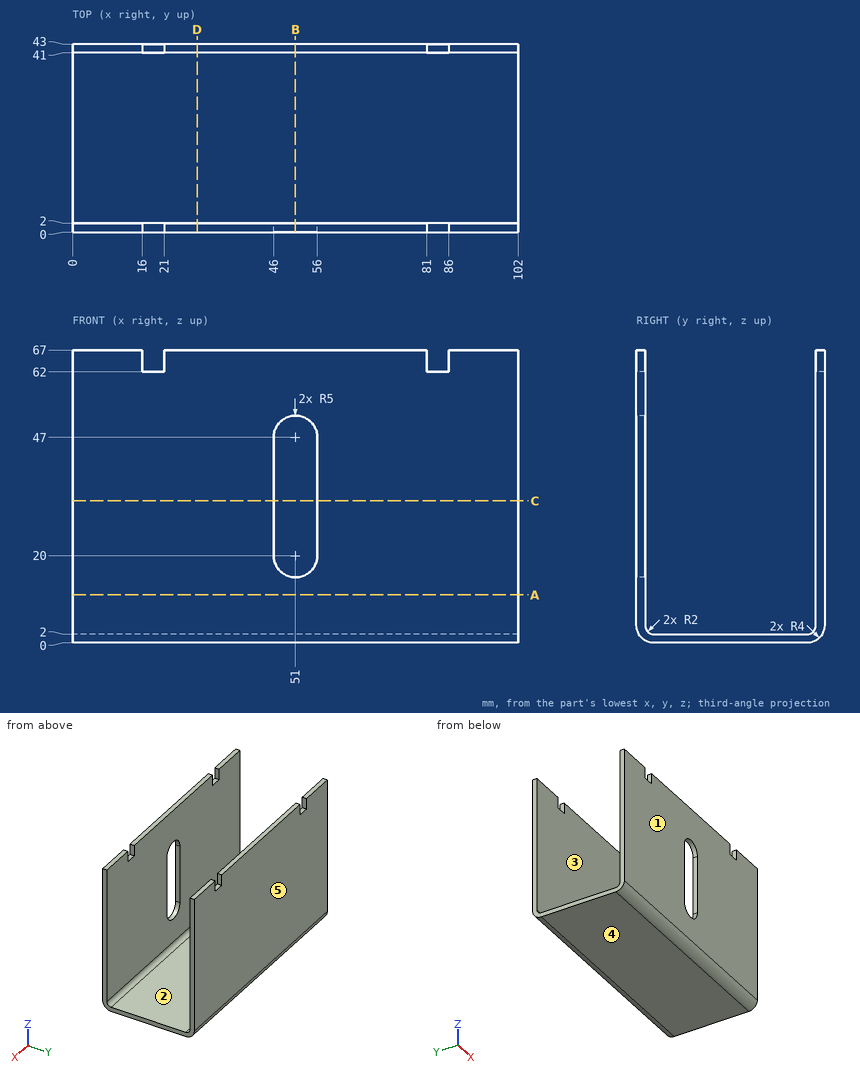
Part print with two shaded views. Sizes in mm from the minimum x, y, z corner. A direction names the side the tool comes from. Coordinates: 2 decimals unless noted, no trailing zeros. Order: outer loops, then holes, each group sorted by start corner. A loop starts at its lowest first (then second) coordinate and runs counter-clockwise, first axis right, second up. Notation, with made-up numbers: (-27.5, 8) - (-6.5, 8) arc R14 ccw to (-6.5, 26) - close; hole circle Ø6 at (-9, -6). An arc over 180 degrees is marked (long way). Answer in a Markdown table with one row per item.
1. Slice it at D-D, the plane x = 28.5. List the corners of the cut face in (y, z).
Answer:
| item | result |
|---|---|
| outline | (0, 4) arc R4 ccw to (4, 0) - (39, 0) arc R4 ccw to (43, 4) - (43, 67) - (41, 67) - (41, 4) arc R2 cw to (39, 2) - (4, 2) arc R2 cw to (2, 4) - (2, 67) - (0, 67) - close |
2. Flat gauge pin, fed straight in: P1, Ø0.6, axis at x = 84, y = 42, coming from the +Z side. Where does the tip first touch, or does it go through?
Answer:
| item | result |
|---|---|
| P1 | z = 62 |
3. Drill centre lines: L1, parallel to Y at x = 67, z = 23; L2, parallel to Z at x = 54, y = 15; L3, parallel to Y at x = 53, z = 28. Where is each one in solid material? Low to high. Write a range as from..to.
Answer:
| item | result |
|---|---|
| L1 | 0..2, 41..43 |
| L2 | 0..2 |
| L3 | 41..43 |
4. Slice it at A-A, the plane z = 11. List the corners of the cut face in (x, y).
Answer:
| item | result |
|---|---|
| outline | (0, 0) - (102, 0) - (102, 2) - (0, 2) - close; (0, 41) - (102, 41) - (102, 43) - (0, 43) - close |
5. Slice it at C-C, the plane z = 32.5. List the corners of the cut face in (x, y), then the cut area to 3 significant figures.
Answer:
| item | result |
|---|---|
| outline | (0, 0) - (46, 0) - (46, 2) - (0, 2) - close; (0, 41) - (102, 41) - (102, 43) - (0, 43) - close; (56, 0) - (102, 0) - (102, 2) - (56, 2) - close |
| area | 388 mm² |
6. Slice it at B-B, the plane x = 51. List the corners of the cut face in (y, z).
Answer:
| item | result |
|---|---|
| outline | (0, 4) arc R4 ccw to (4, 0) - (39, 0) arc R4 ccw to (43, 4) - (43, 67) - (41, 67) - (41, 4) arc R2 cw to (39, 2) - (4, 2) arc R2 cw to (2, 4) - (2, 15) - (0, 15) - close; (0, 52) - (2, 52) - (2, 67) - (0, 67) - close |
7. 3-axis set-ups, long thin cutter, end or side, ignore diameter. For the marked faces 1 and 2: which of +Z, -Z, +X, -X, +Y, -Y reach the whole face in a straight line?
Answer:
| item | result |
|---|---|
| face 1 | +Z, -Z, +X, -X, -Y |
| face 2 | +Z, +X, -X |
8. Pull direction Y, two halves, no side cores. Call the marked faces 3, 4 and 5: +Y half, -Y half, draft (parallel to the pull), parting line (faces both ways), or undercut.
Answer:
| item | result |
|---|---|
| face 3 | undercut |
| face 4 | draft |
| face 5 | +Y half |
